Autodesk Inventor part; units mm, degrees
ref_plane "YZ Plane" through (0, 0, 0) normal (1, 0, 0) x (0, 1, 0)
ref_plane "XZ Plane" through (0, 0, 0) normal (0, 1, 0) x (-1, 0, 0)
ref_plane "XY Plane" through (0, 0, 0) normal (0, 0, 1) x (1, 0, 0)
sketch "Sketch1" plane through (0, 0, 0) normal (0, 1, 0) x (-1, 0, 0)
  line L0 (45, -5) -> (45, -14.75)
  line L1 (45, -14.75) -> (45, -30.25)
  line L2 (45, -30.25) -> (45, -40)
  arc A0 (40, -45) -> (45, -40) centre (40, -40) ccw
  circle A1 centre (40, -40) radius 1.375
  circle A2 centre (40, -5) radius 1.375
  arc A3 (45, -5) -> (40, 0) centre (40, -5) ccw
  line L3 (5, 0) -> (40, 0)
  circle A4 centre (5, -5) radius 1.375
  arc A5 (5, 0) -> (0, -5) centre (5, -5) ccw
  line L4 (0, -14.75) -> (0, -5)
  line L5 (0, -30.25) -> (0, -14.75)
  line L6 (0, -40) -> (0, -30.25)
  arc A6 (0, -40) -> (5, -45) centre (5, -40) ccw
  line L7 (40, -45) -> (5, -45)
  circle A7 centre (5, -40) radius 1.375
  point P0 (0, 0)
  point P1 (0, 0)
extrude "Extrusion1" add sketch "Sketch1" along normal blind 17
sketch "Sketch2" plane through (0, 0, -5) normal (1, 0, 0) x (0, 0, -1)
  line L0 (35, 0) -> (0, 0)
  line L1 (35, 0) -> (35, 17)
  line L2 (0, 17) -> (35, 17)
  line L3 (0, 0) -> (0, 17)
  line L4 (-5, 0) -> (-5, 17)
  line L5 (40, 0) -> (35, 0)
  line L6 (40, 0) -> (40, 17)
  line L7 (35, 17) -> (40, 17)
  line L8 (35, 0) -> (35, 17)
  line L9 (0, 0) -> (-5, 0)
  line L10 (0, 0) -> (0, 17)
  line L11 (-5, 17) -> (0, 17)
  line L12 (-5, 0) -> (-5, 17)
  line L13 (35, 17) -> (0, 17)
  line L14 (0, 0) -> (35, 0)
  line L15 (17.5, 17) -> (25.25, 17)
  line L16 (25.25, 17) -> (9.75, 17)
  line L17 (17.5, 17) -> (17.5, 10.5)
  arc A0 (9.75, 17) -> (25.25, 17) centre (17.5, 18.3702) ccw
  dimension "d8" = 7.75
  dimension "d9" = 15.5
  dimension "d10" = 6.5
extrude "Extrusion2" cut sketch "Sketch2" against normal blind 45 contours A0 L17 L2 | L2 L17 A0
sketch "Sketch3" plane through (-40, 0, 0) normal (0, 0, 1) x (1, 0, 0)
  line L0 (35, 0) -> (0, 0)
  line L1 (35, 0) -> (35, 17)
  line L2 (0, 17) -> (35, 17) construction
  line L3 (0, 0) -> (0, 17)
  line L4 (17.5, 0) -> (9.75, 0)
  line L5 (9.75, 0) -> (25.25, 0)
  line L6 (17.5, 0) -> (17.5, 6.5)
  arc A0 (25.25, 0) -> (9.75, 0) centre (17.5, -1.3702) ccw
  line L7 (35, 0) -> (0, 0)
  point P0 (40, 0)
  point P1 (17.5, 0)
  dimension "d13" = 7.75
  dimension "d14" = 15.5
  dimension "d15" = 6.5
extrude "Extrusion3" cut sketch "Sketch3" against normal blind 45
properties part number "Middle" material "PC/ABS Plastic"
For this review, take the finished solid that the model builds, in its own axes (mm). Round coordinates to 2 decimals unless told otherwise and drop trailing zeros. Loops run counter-clockwise (first coordinate to the right, second up) from the corner with the lowest first, then second, coordinate; pieces in that order, holes last. Notation, with made-up numbers: (38.5, -1.5) - (54.5, -1.5) arc R27 ccw to (54.5, 22.5) - close; hole circle Ø10 at (14, -7). An arc over 180 degrees is marked (long way). Put each result on its own line as item: value. Start each with the question number.
1. Consider section B-B on y = 9.25. State the section outline as (x, z) points (3 decimals).
2. Consider section D-D on x = -22.5. State the section outline as (y, z) points, plus the area to 3 significant figures.
3. For probe 1 along Z at (x, y) = (-5, 8.75) (3 decimals); probe 2 along Z at (x, y) = (-6, 11.5); probe 3 along X at (y, z) = (2.5, -14), list the stretches that pass through material, from the lowest coordinate up. Write a range as [from, to].
4. Mouldability with a two-part tool opening along X and no side actions: class faces 1 (the cylindrical face through (-38.626, 8.381, -5.06)), 2 (the cylindrical face through (-2, 8, -44)), 3 (the flat face through (-22, 8, 0)), 4 (the cylindrical face through (-43, 8, -1)) as +X half, -X half, draft (parallel to the pull), parting line (faces both ways), or undercut.
5. Insertion check: P1, Ø5, axis at x = -19.5, z = -22, coming from the +Y side; P2, Ø8, axis at x = -25, z = -24.5, coming from the +Y side. Each pin has a flat end and moves straight along its axis. Give the tip position at first contact, or say it passes through.
6. Consider section A-A on y = 13. State the section outline as (x, z) points (3 decimals), plus the area to 3 significant figures.
7. Consider section C-C on z = -12.5. State the section outline as (x, y) points.
Result sheet:
1. outline: (-45, -40) arc R5 ccw to (-40, -45) - (-5, -45) arc R5 ccw to (0, -40) - (0, -5) arc R5 ccw to (-5, 0) - (-40, 0) arc R5 ccw to (-45, -5) - close; hole circle Ø2.75 at (-40, -40); hole circle Ø2.75 at (-40, -5); hole circle Ø2.75 at (-5, -40); hole circle Ø2.75 at (-5, -5)
2. outline: (6.5, -45) - (17, -45) - (17, -30.25) arc R7.87 cw to (17, -14.75) - (17, 0) - (6.5, 0) - close
2. area: 397 mm^2
3. probe 1: [-45, -41.375], [-38.625, -6.375], [-3.625, 0]
3. probe 2: [-45, -40.94], [-39.06, -26.34], [-18.66, -5.94], [-4.06, 0]
3. probe 3: [-45, -29.35], [-15.65, 0]
4. face 1: undercut
4. face 2: +X half
4. face 3: draft
4. face 4: -X half
5. P1: y = 11.09
5. P2: y = 13.28
6. outline: (-45, -40) arc R5 ccw to (-40, -45) - (-5, -45) arc R5 ccw to (0, -40) - (0, -28.253) - (-45, -28.253) - close; (-45, -16.747) - (0, -16.747) - (0, -5) arc R5 ccw to (-5, 0) - (-40, 0) arc R5 ccw to (-45, -5) - close; hole circle Ø2.75 at (-40, -40); hole circle Ø2.75 at (-40, -5); hole circle Ø2.75 at (-5, -40); hole circle Ø2.75 at (-5, -5)
6. area: 1,460 mm^2
7. outline: (-45, 0) - (-30.25, 0) arc R7.87 cw to (-14.75, 0) - (0, 0) - (0, 17) - (-45, 17) - close
